Build history of the part. All positions in model axes, mm. A direction names the side the tool comes from. Round coordinates to 2 decimals unless told otherwise and drop trailing zeros. Order: outer loops, then holes, each group sorted by start corner. A loop starts at its lowest first (then second) coordinate and runs counter-clockwise, first axis right, second up. Notation, with made-up numbers: (20.5, 89.25) -> (26.5, 89.25) arc R21 ccw to (26.5, 98.25) -> close; hole circle Ø4 at (-28, 62.5). An arc over 180 degrees is marked (long way). Answer as a JSON object with one key per item and string values.
from build123d import *

# Parameters (mm, degrees)
SKETCH1_R           = 1
BOSS_EXTRUDE1_DEPTH = 3.5


with BuildPart() as part:
    # Sketch1 → Boss-Extrude1 (new body)
    with BuildSketch(Plane.XY):
        with BuildLine():
            Line((0, 0), (0, 13))
            ThreePointArc((0, 13), (0.585786438, 14.414213562), (2, 15))
            Line((2, 15), (23.872983346, 15))
            ThreePointArc((23.872983346, 15), (31.372983346, 7.5), (23.872983346, 0))
            Line((23.872983346, 0), (18.455559041, 0))
            ThreePointArc((18.455559041, 0), (17.360113926, -0.326679947), (16.622528763, -1.2))
            ThreePointArc((16.622528763, -1.2), (13.872983346, -3), (11.123437929, -1.2))
            ThreePointArc((11.123437929, -1.2), (10.385852766, -0.326679947), (9.290407651, 0))
            Line((9.290407651, 0), (0, 0))
        make_face()
        with Locations((3.872983346, 7.5)):
            Circle(SKETCH1_R, mode=Mode.SUBTRACT)
        with Locations((23.872983346, 7.5)):
            Circle(SKETCH1_R, mode=Mode.SUBTRACT)
        with Locations((13.872983346, 0)):
            Circle(SKETCH1_R, mode=Mode.SUBTRACT)
        with Locations((3.872983346, 2.5)):
            Circle(SKETCH1_R, mode=Mode.SUBTRACT)
    extrude(amount=BOSS_EXTRUDE1_DEPTH)


solid = part.part
1) Cut at D-D, the plane y = 2.5. Give the cut face in (x, z).
Checked values:
{"outline": "(0, 0) -> (2.87, 0) -> (2.87, 3.5) -> (0, 3.5) -> close; (4.87, 0) -> (29.46, 0) -> (29.46, 3.5) -> (4.87, 3.5) -> close"}
2) Flat gauge pins, fed straight in: pin 1 Ø1.8 at (x, z) = (22, 1.5) entering from -Y; pin 2 Ø1.6 at (x, y) = (3.87, 7.5) entering from +Z. Where does each tip first touch, or does it go through?
Checked values:
{"pin 1": "stops at y = 0", "pin 2": "passes through"}
3) Cut at B-B, the plane z = 3.05. Give the cut face in (x, y).
Checked values:
{"outline": "(0, 0) -> (9.29, 0) arc R2 cw to (11.12, -1.2) arc R3 ccw to (16.62, -1.2) arc R2 cw to (18.46, 0) -> (23.87, 0) arc R7.5 ccw to (23.87, 15) -> (2, 15) arc R2 ccw to (0, 13) -> close; hole circle Ø2 at (3.87, 2.5); hole circle Ø2 at (3.87, 7.5); hole circle Ø2 at (13.87, 0); hole circle Ø2 at (23.87, 7.5)"}
4) Pull direction X, two halves, no side cores. Call faces 1 (the face through (21, 0, 2)), 2 (the face through (10.399, -0.336, 1.726)), 3 (the face through (3.74, 3.49, 1.73)): pulls with the +X half, pulls with the -X half, needs draft (parallel to the pull), parting line crosses it, or undercut.
Checked values:
{"face 1": "needs draft", "face 2": "pulls with the -X half", "face 3": "undercut"}
5) Cut at A-A, the plane y = 7.5. Give the cut face in (x, z), plus the area to 3 significant figures.
Checked values:
{"outline": "(0, 0) -> (2.87, 0) -> (2.87, 3.5) -> (0, 3.5) -> close; (4.87, 0) -> (22.87, 0) -> (22.87, 3.5) -> (4.87, 3.5) -> close; (24.87, 0) -> (31.37, 0) -> (31.37, 3.5) -> (24.87, 3.5) -> close", "area": "95.8 mm²"}
6) Probe L1, parallel to Y at x = 14, z = 1.6; L2, parallel to Y at x = 23, z = 1.75; L3, parallel to Y at x = 8, z = 1.7. List the from-to ranges inside material, lowest first. Write a range as from..to.
Checked values:
{"L1": "y = -3..-0.99, 0.99..15", "L2": "y = 0..7.01, 7.99..15", "L3": "y = 0..15"}
7) Which spindle directions (+Z, -Z, +X, -X, +Y, -Y) get a long thin tool onto all of the face, cutting with end or side? Do faces 4 (the face through (5, 0, 2)), 5 (the face through (23.14, 8.18, 1.73)). Say none if no direction does.
Checked values:
{"face 4": "+Z, -Z, -X, -Y", "face 5": "+Z, -Z"}
8) Cut at C-C, the plane x = 23.5. Give the cut face in (y, z), plus the area to 3 significant figures.
Checked values:
{"outline": "(0, 0) -> (6.57, 0) -> (6.57, 3.5) -> (0, 3.5) -> close; (8.43, 0) -> (15, 0) -> (15, 3.5) -> (8.43, 3.5) -> close", "area": "46.0 mm²"}
